Geometry: see drawing. Coordinates: mm, zero at the bounding-box minimum. A direction names the side the tool comes from. Give positions to 0.01 mm unless a question says otherwise; leave off trailing zeros. Write each loop counter-clockwise with the first axis right and the second up, starting at its lowest first coordinate (ties: lowest second). Pieces come first, ordered by that corner, then holes. Notation, with made-up numbers: (36.5, -15.75) - (63.5, -15.75) arc R19 cw to (63.5, 5.25) - close; hole circle Ø1 at (-7, 77). An arc over 180 degrees is marked (long way). Return JSON: item names as keys, results as strings.
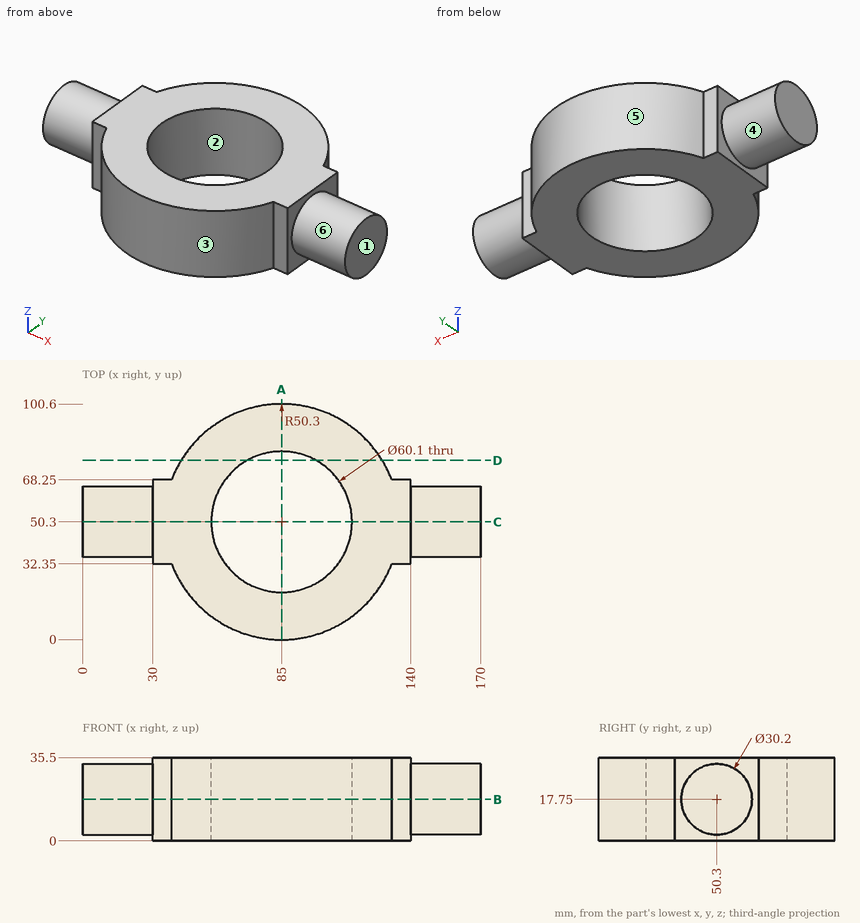
Q1. Section query C-C, the plane y = 50.3. Return the cut outline in (x, z).
Answer key:
{"outline": "(0, 2.65) - (30, 2.65) - (30, 0) - (54.95, 0) - (54.95, 35.5) - (30, 35.5) - (30, 32.85) - (0, 32.85) - close; (115.05, 0) - (140, 0) - (140, 2.65) - (170, 2.65) - (170, 32.85) - (140, 32.85) - (140, 35.5) - (115.05, 35.5) - close"}
Q2. Section query B-B, the plane z = 17.75. Return the cut outline in (x, y).
Answer key:
{"outline": "(0, 35.2) - (30, 35.2) - (30, 32.35) - (38.01, 32.35) arc R50.3 ccw to (131.99, 32.35) - (140, 32.35) - (140, 35.2) - (170, 35.2) - (170, 65.4) - (140, 65.4) - (140, 68.25) - (131.99, 68.25) arc R50.3 ccw to (38.01, 68.25) - (30, 68.25) - (30, 65.4) - (0, 65.4) - close; hole circle Ø60.1 at (85, 50.3)"}
Q3. Set-up query: the marked faces 4, 5 and 6. Return all of +Z, -Z, +X, -X, +Y, -Y with unobstructed straight access to the full face (end or side cutting, diameter ignored); none if empty.
Answer key:
{"face 4": "-X", "face 5": "+Z, -Z, +Y", "face 6": "+X"}
Q4. Section query A-A, the plane x = 85. Return the cut outline in (y, z), plus the area to 3 significant figures.
Answer key:
{"outline": "(0, 0) - (20.25, 0) - (20.25, 35.5) - (0, 35.5) - close; (80.35, 0) - (100.6, 0) - (100.6, 35.5) - (80.35, 35.5) - close", "area": "1,440 mm^2"}
Q5. Pin query (flat end, axial travel): P1, Ø9, axis at x = 136, z = 19, coming from the +Y side; P2, Ø1, axis at x = 46, z = 6.5, coming from the +Y side; P3, Ø6.5, axis at x = 36, z = 14, coming from the +Y side. Return the tip coordinate at first contact, or that it passes through.
Answer key:
{"P1": "stops at y = 69.48", "P2": "stops at y = 82.67", "P3": "stops at y = 71.21"}
Q6. Material intervals for probe 1 along Y at (x, z) = (85, 16); probe 2 along X at (y, z) = (50, 19); probe 3 along Y at (x, z) = (90.5, 7), sorted ascending. Write a range as [from, to].
Answer key:
{"probe 1": "y = [0, 20.25], [80.35, 100.6]", "probe 2": "x = [0, 54.95], [115.05, 170]", "probe 3": "y = [0.3, 20.76], [79.84, 100.3]"}
Q7. Mould query, pull axis Y, two halves, no side actions, for the marked faces 1, 2 and 3. Classes: pulls with the +Y half, pulls with the -Y half, needs draft (parallel to the pull), parting line crosses it, or undercut.
Answer key:
{"face 1": "needs draft", "face 2": "undercut", "face 3": "pulls with the -Y half"}
Q8. Section query D-D, the plane y = 76.5. Return the cut outline in (x, z), plus the area to 3 significant figures.
Answer key:
{"outline": "(42.06, 0) - (70.28, 0) - (70.28, 35.5) - (42.06, 35.5) - close; (99.72, 0) - (127.94, 0) - (127.94, 35.5) - (99.72, 35.5) - close", "area": "2,000 mm^2"}
